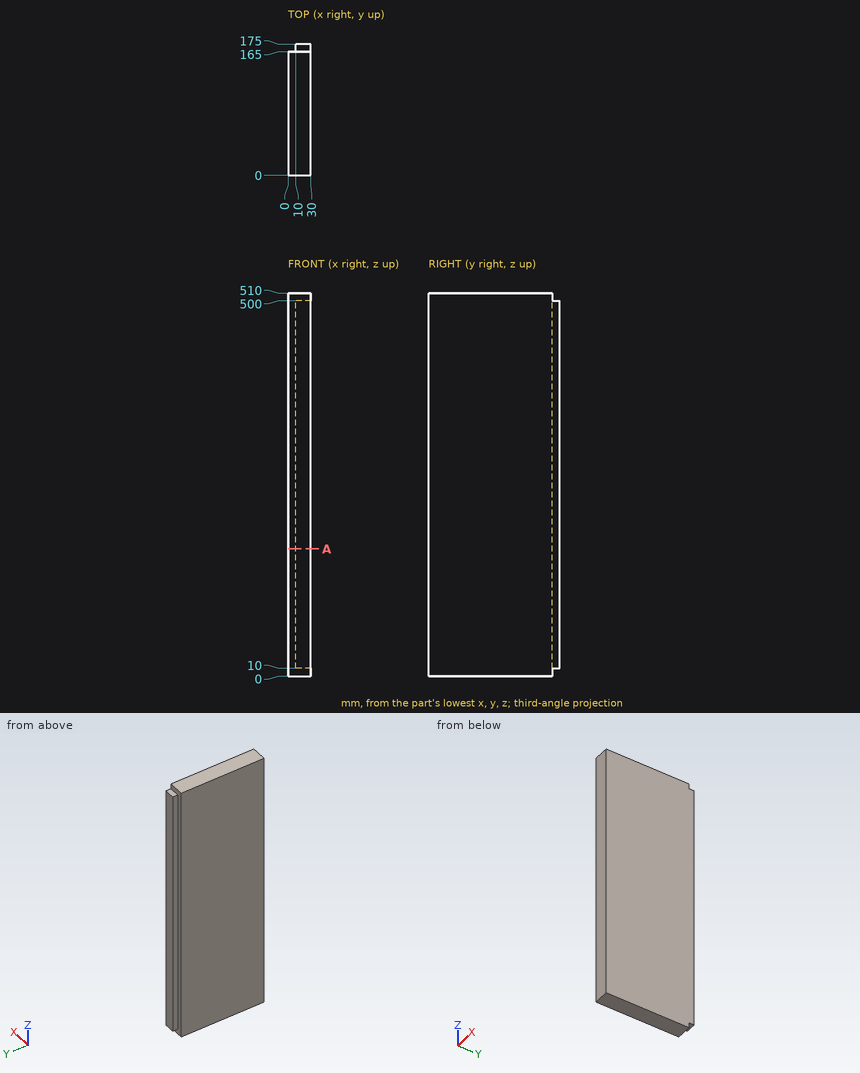
Geometry: see drawing. Coordinates: mm, zero at the bounding-box minimum. Coordinates: 2 decimals unless noted, no trailing zeros. Loops run counter-clockwise (first coordinate to the right, second up) from the corner with the lowest first, then second, coordinate; pieces in that order, holes last. Notation, with made-up numbers: (75.5, 14) - (92.5, 14) arc R17 cw to (92.5, 20) - close; hole circle Ø5 at (21, 60.25). An arc over 180 degrees is marked (long way). Return JSON: item names as keys, results as strings.
Q1. Section A-A, the plane z = 169.5. Return loops of the section in (x, y), plus the area to 3 significant figures.
Results:
{"outline": "(0, 0) - (30, 0) - (30, 175) - (10, 175) - (10, 165) - (0, 165) - close", "area": "5,150 mm2"}
Q2. Material intervals for line 1 along Y through (x, z) = (3.5, 404), sorted ascending.
Results:
{"line 1": "0 to 165"}
Q3. Contact query for flat-ended pins moving along their axis: P1, Ø8, axis at y = 172.5, z = 220, coming from the -X side; P2, Ø8, axis at x = 24.5, y = 169.5, coming from the +Z side. Output: stop coordinate, or through.
Results:
{"P1": "x = 10", "P2": "z = 500"}
